Can you work these out from the model? Positions are in its coordinate system, mm. A direction names the side the tool comes from. Round coordinates to 2 decimals unless told otherwise and drop trailing zeros. Write each loop counter-clockwise with the first axis right and the second up, starting at its lowest first coordinate (ties: lowest second). Pieces come first, ordered by that corner, then holes. Notation, with made-up numbers: (19, 51.25) -> (36, 51.25) arc R27 cw to (36, 72.25) -> close; hole circle Ø9 at (42, -17). An arc over 180 degrees is marked (long way). Use CSV: the item, a comma, the result in double quotes.
```python
from build123d import *


with BuildPart() as f2:
    # F2: sweep along a path in F0
    with BuildLine(Plane.XY) as f2_path:
        Line((0, 0), (2438.4, 0))
        Line((2438.4, 0), (2438.4, 1170))
        Line((2438.4, 1170), (0, 1170))
        Line((0, 1170), (0, 0))
    # F1 (on Right) → F2 (sweep)
    with BuildSketch(Plane.YZ):
        Polygon((38.1, 0), (0, 0), (0, -76.2), (38.1, -76.2), (38.1, -71.12), (6.35, -66.2), (6.35, -10), (38.1, -5.08), align=None)
    sweep(path=f2_path.line, transition=Transition.RIGHT)


solid = f2.part
```
Q1. Suppose I cut it at C-C (x = 1093). Write out the boundary of the cut face in (y, z).
Resolved:
outline,"(0, -76.2) -> (38.1, -76.2) -> (38.1, -71.12) -> (6.35, -66.2) -> (6.35, -10) -> (38.1, -5.08) -> (38.1, 0) -> (0, 0) -> close; (1131.9, -76.2) -> (1170, -76.2) -> (1170, 0) -> (1131.9, 0) -> (1131.9, -5.08) -> (1163.65, -10) -> (1163.65, -66.2) -> (1131.9, -71.12) -> close"
Q2. Will this pin go through, and if not, where does the flat tip stop? P1, Ø1.5, axis at x = 1614.5, z = -1.5, coming from the -Y side.
Resolved:
P1,"stops at y = 0"
Q3. Suppose I cut it at A-A (z = -44.5). Write out the boundary of the cut face in (x, y), and give its area (3 significant figures).
Resolved:
outline,"(0, 0) -> (2438.4, 0) -> (2438.4, 1170) -> (0, 1170) -> close; hole (6.35, 6.35) -> (2432.05, 6.35) -> (2432.05, 1163.65) -> (6.35, 1163.65) -> close"
area,"45,700 mm^2"
Q4. If we mould it in two halves opening along Z, with no side actions, what happens to faces 3 (the face through (1225, 1151, 0)), 4 (the face through (1202, 1163.65, -38)), 5 (the face through (1202, 1170, -38))? For each: released by +Z, released by -Z, zero draft, split by the parting line, or undercut.
Resolved:
face 3,"released by +Z"
face 4,"undercut"
face 5,"zero draft"
Q5. Suppose I cut it at B-B (y = 720.5). Write out the boundary of the cut face in (x, z).
Resolved:
outline,"(0, -76.2) -> (38.1, -76.2) -> (38.1, -71.12) -> (6.35, -66.2) -> (6.35, -10) -> (38.1, -5.08) -> (38.1, 0) -> (0, 0) -> close; (2400.3, -76.2) -> (2438.4, -76.2) -> (2438.4, 0) -> (2400.3, 0) -> (2400.3, -5.08) -> (2432.05, -10) -> (2432.05, -66.2) -> (2400.3, -71.12) -> close"
Q6. On a 3-axis mill with a long thin cutter (end or side, diameter ignored), from which of +Z, -Z, +X, -X, +Y, -Y can I reach the whole of each face in a straight line? I mean faces 1 (the face through (6.35, 577, -38)), 2 (the face through (0, 577, -38)). Say none if no direction works.
Resolved:
face 1,"none"
face 2,"+Z, -Z, -X, +Y, -Y"
Q7. Please list where these lines run through material, in increasing order: probe 1 along Y at (x, z) = (1999.5, -51); probe 2 along X at (y, z) = (712.5, -21); probe 3 along Y at (x, z) = (402.5, -4).
Resolved:
probe 1,"y = 0 to 6.35, 1163.65 to 1170"
probe 2,"x = 0 to 6.35, 2432.05 to 2438.4"
probe 3,"y = 0 to 38.1, 1131.9 to 1170"
